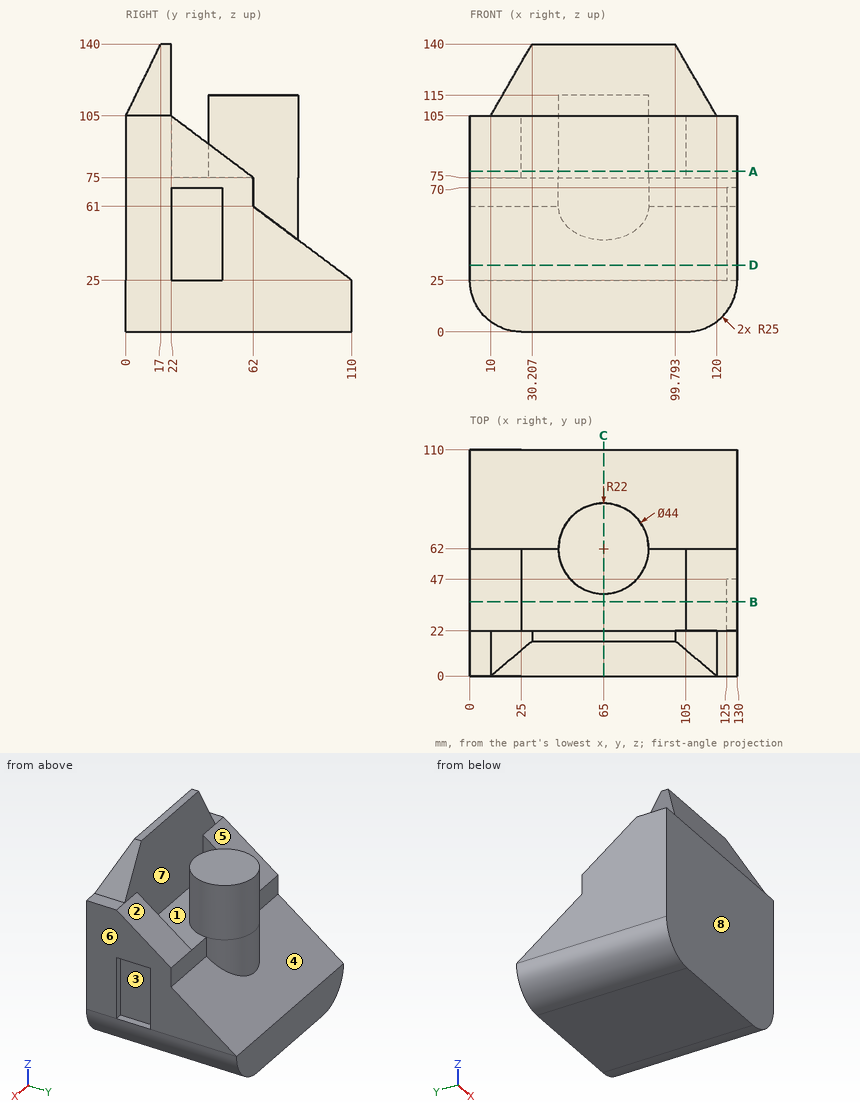
The drawing under review shows one solid part. Ordinate dimensions are in mm from its lowest x, y, z. A direction names the side the tool comes from. Coordinates: 2 decimals unless noted, no trailing zeros. Order: outer loops, then holes, each group sorted by start corner. A loop starts at its lowest first (then second) coordinate and runs counter-clockwise, first axis right, second up. Notation, with made-up numbers: (-15, 36.25) -> (1, 36.25) arc R10 ccw to (1, 51.25) -> close; hole circle Ø5 at (21.5, 77). An arc over 180 degrees is marked (long way). Answer in a Markdown table with one row per item. Add a question column.
Item 1: We need section B-B on y = 36. Write out the cut boundary in (x, z), plus the area to 3 significant figures.
Item 2: Machinability: for the marked faces 1, 2, 3 and 4, which of the approach directions +Z, -Z, +X, -X, +Y, -Y give a long, thin tool a straight path to every point of the face, cutting with its end or side? Answer none if there is none.
Item 3: We need section C-C on x = 65. Write out the cut boundary in (y, z), plus the area to 3 significant figures.
Item 4: To check wall thickness, follow probe 1 along Y at (x, z) = (103.5, 79.5); probe 2 along X at (y, z) = (29, 82.5); probe 3 along Z at (x, y) = (38, 35). State the ranges of each line that lie inside material, in increasing order.
Item 5: Clearance check with flat-ended pins moving along their axes: pin 1 (3 mm diameter, centred on y = 78.5, z = 61.5, fed in from -X); pin 2 (8 mm diameter, centred on x = 5.5, y = 10, fed in from +Z); pin 3 (4 mm diameter, centred on x = 27, z = 67.5, fed in from +Y); pin 4 (6 mm diameter, centred on x = 104, y = 89, fed in from -Z). State where each tip first meets the part, or that it passes through.
Item 6: Mouldability with a two-part tool opening along Y and no side actions: class the marked faces 5, 6, 7 and 8 as +Y half, -Y half, draft (parallel to the pull), parting line (faces both ways), or undercut.
Item 7: We need section A-A on z = 78. Write out the cut boundary in (x, y), plus the area to 3 significant figures.
Item 8: We need section D-D on z = 32.5. Write out the cut boundary in (x, y), plus the area to 3 significant figures.
Final values:
| question | item | result |
|---|---|---|
| 1 | outline | (0, 25) arc R25 ccw to (25, 0) -> (105, 0) arc R25 ccw to (130, 25) -> (125, 25) -> (125, 70) -> (130, 70) -> (130, 94.5) -> (105, 94.5) -> (105, 75) -> (25, 75) -> (25, 94.5) -> (0, 94.5) -> close |
| 1 | area | 10,200 mm2 |
| 2 | face 1 | +Z |
| 2 | face 2 | +Z, +X, +Y |
| 2 | face 3 | +X |
| 2 | face 4 | +Z, +Y |
| 3 | outline | (0, 0) -> (110, 0) -> (110, 25) -> (84, 44.5) -> (84, 115) -> (40, 115) -> (40, 75) -> (22, 75) -> (22, 140) -> (17, 140) -> (0, 105) -> close |
| 3 | area | 10,100 mm2 |
| 4 | probe 1 | y = 0 to 22 |
| 4 | probe 2 | x = 0 to 25, 105 to 130 |
| 4 | probe 3 | z = 0 to 75 |
| 5 | pin 1 | stops at x = 48.91 |
| 5 | pin 2 | stops at z = 105 |
| 5 | pin 3 | stops at y = 62 |
| 5 | pin 4 | stops at z = 0 |
| 6 | face 5 | +Y half |
| 6 | face 6 | draft |
| 6 | face 7 | undercut |
| 6 | face 8 | -Y half |
| 7 | outline | (0, 0) -> (130, 0) -> (130, 58) -> (105, 58) -> (105, 22) -> (25, 22) -> (25, 58) -> (0, 58) -> close; circle Ø44 at (65, 62) |
| 7 | area | 6,180 mm2 |
| 8 | outline | (0, 0) -> (130, 0) -> (130, 22) -> (125, 22) -> (125, 47) -> (130, 47) -> (130, 100) -> (0, 100) -> close |
| 8 | area | 12,900 mm2 |
